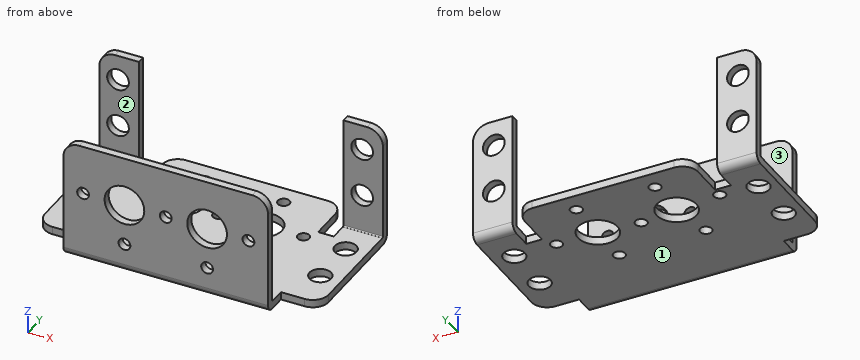
from build123d import *

# Parameters (mm, degrees)
SKETCH1_R      = 4.0005
SKETCH1_R_2    = 1.1938
SKETCH1_R_3    = 2.1844
EXTRUDE2_DEPTH = 1.5748
SKETCH3_W      = 7.9502
SKETCH3_H      = 1.5748
SKETCH3_W_2    = 41.2496
EXTRUDE3_DEPTH = 22.6314
FILLET1_R      = 3.175
FILLET2_R      = 1.5748
FILLET3_R      = 0.254
SKETCH4_R      = 4.0005
SKETCH4_R_2    = 1.1938
EXTRUDE4_DEPTH = 1.5748
SKETCH5_R      = 2.1844
EXTRUDE5_DEPTH = 1.5748


with BuildPart() as part:
    # Sketch1 → Extrude2 (new body)
    with BuildSketch(Plane.XY):
        with BuildLine():
            Line((11.9126, 30.734), (11.9126, 32.041994716))
            ThreePointArc((11.9126, 32.041994716), (12.84253597, 34.287058746), (15.0876, 35.216994716))
            Line((15.0876, 35.216994716), (43.6626, 35.216994716))
            ThreePointArc((43.6626, 35.216994716), (45.90766403, 34.287058746), (46.8376, 32.041994716))
            Line((46.8376, 32.041994716), (46.8376, 30.734))
            Line((46.8376, 30.734), (46.8376, 25.4))
            Line((46.8376, 25.4), (49.9872, 25.4))
            Line((49.9872, 25.4), (49.9872, 30.734))
            Line((49.9872, 30.734), (57.9374, 30.734))
            Line((57.9374, 30.734), (57.9374, 8.128))
            ThreePointArc((57.9374, 8.128), (57.00746403, 5.88293597), (54.7624, 4.953))
            Line((54.7624, 4.953), (49.9872, 4.953))
            Line((49.9872, 4.953), (49.9872, 0))
            Line((49.9872, 0), (8.7376, 0))
            Line((8.7376, 0), (8.7376, 4.953))
            Line((8.7376, 4.953), (3.9624, 4.953))
            ThreePointArc((3.9624, 4.953), (1.71733597, 5.88293597), (0.7874, 8.128))
            Line((0.7874, 8.128), (0.7874, 30.734))
            Line((0.7874, 30.734), (8.7376, 30.734))
            Line((8.7376, 30.734), (8.7376, 25.4))
            Line((8.7376, 25.4), (11.9126, 25.4))
            Line((11.9126, 25.4), (11.9126, 30.734))
        make_face()
        with Locations((21.0312, 22.8092)):
            Circle(SKETCH1_R, mode=Mode.SUBTRACT)
        with Locations((21.0312, 31.1404)):
            Circle(SKETCH1_R_2, mode=Mode.SUBTRACT)
        with Locations((28.575, 22.0218)):
            Circle(SKETCH1_R_2, mode=Mode.SUBTRACT)
        with Locations((19.4564, 14.478)):
            Circle(SKETCH1_R_2, mode=Mode.SUBTRACT)
        with Locations((11.9126, 23.5966)):
            Circle(SKETCH1_R_2, mode=Mode.SUBTRACT)
        with Locations((36.9062, 31.1404)):
            Circle(SKETCH1_R_2, mode=Mode.SUBTRACT)
        with Locations((45.2374, 22.8092)):
            Circle(SKETCH1_R_2, mode=Mode.SUBTRACT)
        with Locations((36.9062, 22.8092)):
            Circle(SKETCH1_R, mode=Mode.SUBTRACT)
        with Locations((36.9062, 14.478)):
            Circle(SKETCH1_R_2, mode=Mode.SUBTRACT)
        with Locations((4.5466, 22.7838)):
            Circle(SKETCH1_R_3, mode=Mode.SUBTRACT)
        with Locations((4.5466, 12.9794)):
            Circle(SKETCH1_R_3, mode=Mode.SUBTRACT)
        with Locations((53.7464, 22.7838)):
            Circle(SKETCH1_R_3, mode=Mode.SUBTRACT)
        with Locations((53.7464, 12.9794)):
            Circle(SKETCH1_R_3, mode=Mode.SUBTRACT)
    extrude(amount=EXTRUDE2_DEPTH)

    # Sketch3 → Extrude3 (add)
    with BuildSketch(Plane.XY.offset(1.5748)):
        with Locations((4.7625, 29.9466)):
            Rectangle(SKETCH3_W, SKETCH3_H)
        with Locations((29.3624, 0.7874)):
            Rectangle(SKETCH3_W_2, SKETCH3_H)
        with Locations((53.9623, 29.9466)):
            Rectangle(SKETCH3_W, SKETCH3_H)
    extrude(amount=EXTRUDE3_DEPTH)

    # Fillet1
    fillet1_edges = [part.edges().sort_by_distance(p)[0] for p in [
        (0.7874, 29.9466, 24.2062),
        (8.7376, 0.7874, 24.2062),
        (49.9872, 0.7874, 24.2062),
        (57.9374, 29.9466, 24.2062),
    ]]
    fillet(fillet1_edges, radius=FILLET1_R)

    # Fillet2
    fillet2_edges = [part.edges().sort_by_distance(p)[0] for p in [
        (4.7625, 30.734, 0),
        (53.9623, 30.734, 0),
        (29.3624, 0, 0),
    ]]
    fillet(fillet2_edges, radius=FILLET2_R)

    # Fillet3
    fillet3_edges = [part.edges().sort_by_distance(p)[0] for p in [
        (4.7625, 29.1592, 1.5748),
        (29.3624, 1.5748, 1.5748),
        (53.9623, 29.1592, 1.5748),
    ]]
    fillet(fillet3_edges, radius=FILLET3_R)

    # Sketch4 → Extrude4 (cut)
    with BuildSketch(Plane.XZ):
        with Locations(Location((21.0312, 14.2494, 0), (0, 0, 270))):  # turned: the seam where the file's is
            Circle(SKETCH4_R)
        with Locations(Location((12.7, 14.2494, 0), (0, 0, 270))):  # turned: the seam where the file's is
            Circle(SKETCH4_R_2)
        with Locations(Location((21.0312, 5.9182, 0), (0, 0, 270))):  # turned: the seam where the file's is
            Circle(SKETCH4_R_2)
        with Locations(Location((29.3624, 14.2494, 0), (0, 0, 270))):  # turned: the seam where the file's is
            Circle(SKETCH4_R_2)
        with Locations(Location((46.0248, 14.2494, 0), (0, 0, 270))):  # turned: the seam where the file's is
            Circle(SKETCH4_R_2)
        with Locations(Location((37.6936, 14.2494, 0), (0, 0, 270))):  # turned: the seam where the file's is
            Circle(SKETCH4_R)
        with Locations(Location((37.6936, 5.9182, 0), (0, 0, 270))):  # turned: the seam where the file's is
            Circle(SKETCH4_R_2)
    extrude(amount=-EXTRUDE4_DEPTH, mode=Mode.SUBTRACT)

    # Sketch5 → Extrude5 (cut)
    with BuildSketch(Plane(origin=(0, 30.734, 0), x_dir=(1, 0, 0), z_dir=(0, 1, 0))):
        with Locations(Location((4.5466, -9.3218, 0), (0, 0, 270))):  # turned: the seam where the file's is
            Circle(SKETCH5_R)
        with Locations(Location((4.5466, -19.1262, 0), (0, 0, 270))):  # turned: the seam where the file's is
            Circle(SKETCH5_R)
        with Locations(Location((53.7464, -19.1262, 0), (0, 0, 270))):  # turned: the seam where the file's is
            Circle(SKETCH5_R)
        with Locations(Location((53.7464, -9.3218, 0), (0, 0, 270))):  # turned: the seam where the file's is
            Circle(SKETCH5_R)
    extrude(amount=-EXTRUDE5_DEPTH, mode=Mode.SUBTRACT)


solid = part.part
Could you check a few things on this model? Use its own coordinates, in mm. Face numbers are marked on the shaded views. A direction names the side the tool comes from. Give positions to 0.01 mm unless a question says otherwise; leave off trailing zeros. Write each loop counter-clockwise with the first axis right and the second up, starting at its lowest first coordinate (ties: lowest second). Pieces come first, ordered by that corner, then holes. Notation, with made-up numbers: (36.25, -18) - (85.25, -18) arc R15 ccw to (85.25, 2) - close; hole circle Ø9 at (30, -33.75). An arc over 180 degrees is marked (long way). Use CSV: the item, a comma, the result in double quotes. Start each with the question number.
Item 1: For the marked faces 1, 2 and 3, which set-ups out of +Z, -Z, +X, -X, +Y, -Y let a thin tool reach every point of the face, with its end or its side?
Item 2: I want a section at D-D, the plane z = 7.75. Please give me the cut outline in (x, y), then the cut area to 3 significant figures.
Item 3: I want a section at A-A, the plane x = 31.5. Please give me the cut outline in (y, z).
Item 4: I want a section at B-B, the plane z = 19.75. Please give me the cut outline in (x, y).
Item 5: If I drill on line 1 along X through (y, z) = (30, 3); line 2 along Y through (x, z) = (31, 12.5); line 3 along Y through (x, z) = (18.5, 1.25), over which ranges is the centre line in solid material (lowest first)?
Item 6: I'm going to push flat-ended pins straight in: pin 1 (3 mm diameter, centred on x = 47, y = 28, fed in from -Z); pin 2 (1 mm diameter, centred on x = 8.5, y = 28.5, fed in from +Z); pin 3 (4 mm diameter, centred on x = 36.5, z = 5.5, fed in from +Y); pin 4 (8 mm diameter, centred on x = 51.5, z = 14.5, fed in from +Y). Where does each tip first touch, or does it pass through?
Item 7: I want a section at C-C, the plane y = 3. Please give me the cut outline in (x, z).
Findings:
1,face 1,"-Z, +X, -X, +Y, -Y"
1,face 2,"+Z, +X, -X, -Y"
1,face 3,"+Z, +X, -X, +Y"
2,outline,"(0.79, 29.16) - (3.03, 29.16) - (3.03, 30.73) - (0.79, 30.73) - close; (6.06, 29.16) - (8.74, 29.16) - (8.74, 30.73) - (6.06, 30.73) - close; (8.74, 0) - (49.99, 0) - (49.99, 1.57) - (8.74, 1.57) - close; (49.99, 29.16) - (52.23, 29.16) - (52.23, 30.73) - (49.99, 30.73) - close; (55.26, 29.16) - (57.94, 29.16) - (57.94, 30.73) - (55.26, 30.73) - close"
2,area,"80.4 mm2"
3,outline,"(0, 1.57) arc R1.57 ccw to (1.57, 0) - (35.22, 0) - (35.22, 1.57) - (1.83, 1.57) arc R0.25 cw to (1.57, 1.83) - (1.57, 24.21) - (0, 24.21) - close"
4,outline,"(0.79, 29.16) - (2.45, 29.16) - (2.45, 30.73) - (0.79, 30.73) - close; (6.64, 29.16) - (8.74, 29.16) - (8.74, 30.73) - (6.64, 30.73) - close; (8.74, 0) - (49.99, 0) - (49.99, 1.57) - (8.74, 1.57) - close; (49.99, 29.16) - (51.65, 29.16) - (51.65, 30.73) - (49.99, 30.73) - close; (55.84, 29.16) - (57.94, 29.16) - (57.94, 30.73) - (55.84, 30.73) - close"
5,line 1,"x = 0.79 to 8.74, 49.99 to 57.94"
5,line 2,"y = 0 to 1.57"
5,line 3,"y = 0.03 to 13.76, 15.19 to 19.71, 25.91 to 35.22"
6,pin 1,"stops at z = 0"
6,pin 2,"stops at z = 1.59"
6,pin 3,"stops at y = 1.57"
6,pin 4,"stops at y = 30.73"
7,outline,"(8.74, 0) - (49.99, 0) - (49.99, 1.57) - (8.74, 1.57) - close"
